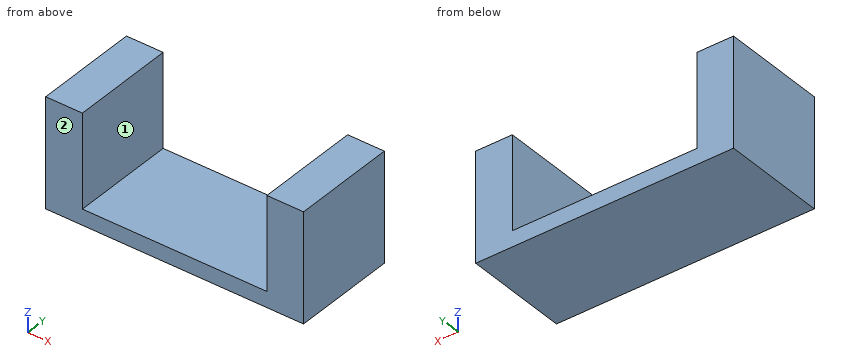
```python
from build123d import *

# Parameters (mm, degrees)
F0_W     = 54.864
F0_H     = 25.4
F1_DEPTH = 3.81
F2_W     = 5.08
F2_H     = 25.4
F3_DEPTH = 22.606
F5_W     = 25.4
F5_H     = 22.606
F5_H_2   = 3.81
F6_DEPTH = 3.81
F4_W     = 25.4
F4_H     = 3.81
F4_H_2   = 22.606
F7_DEPTH = 3.81


with BuildPart() as f1:
    # F0 (on Top) → F1 (new body)
    with BuildSketch(Plane.XY):
        Rectangle(F0_W, F0_H)
    extrude(amount=F1_DEPTH)

    # F2 (on face) → F3 (join)
    with BuildSketch(Plane.XY.offset(3.81)):
        with Locations((-24.892, 0)):
            Rectangle(F2_W, F2_H)
        with Locations((24.892, 0)):
            Rectangle(F2_W, F2_H)
    extrude(amount=F3_DEPTH)

    # F5 (on face) → F6 (join)
    with BuildSketch(Plane.YZ.offset(27.432)):
        with Locations((0, 11.303)):
            Rectangle(F5_W, F5_H)
        with Locations((0, 24.511)):
            Rectangle(F5_W, F5_H_2)
    extrude(amount=F6_DEPTH)

    # F4 (on face) → F7 (join)
    with BuildSketch(Plane(origin=(-27.432, 0, 0), x_dir=(0, -1, 0), z_dir=(-1, 0, 0))):
        with Locations((0, 24.511)):
            Rectangle(F4_W, F4_H)
        with Locations((0, 11.303)):
            Rectangle(F4_W, F4_H_2)
    extrude(amount=F7_DEPTH)


solid = f1.part
```
Check sheet for the modelled part. Datum: model origin and axes. Units: mm. Face numbers are marked on the shaded views. A direction names the side the tool comes from. Coordinates: 2 decimals unless noted, no trailing zeros. Loops run counter-clockwise (first coordinate to the right, second up) from the corner with the lowest first, then second, coordinate; pieces in that order, holes last. Notation, with made-up numbers: M -28.75,60.25 L -1.75,60.25 A31 ccw -1.75,88.25 Z; hole C 58,13 d8. An arc over 180 degrees is marked long. Answer as a JSON object with one key per item and string values.
1. Scan lines: L1, parallel to X at y = -5.75, z = 18; L2, parallel to Z at x = -16.5, y = 7. Record each from-to range of solid material in increasing order. Write a range as from..to.
Outcome:
{"L1": "-31.24..-22.35, 22.35..31.24", "L2": "0..3.81"}
2. Access from +Z, -Z, +X, -X, +Y, -Y to the whole of each face (thin tool, end or side, straight path). Record for the marked faces 1 and 2.
Outcome:
{"face 1": "+Z, +Y, -Y", "face 2": "+Z, -Z, +X, -X, -Y"}
3. Sectioned sample at A-A on z = 8. Record the cut outline in (x, y), and give its area (3 significant figures).
Outcome:
{"outline": "M -31.24,-12.7 L -22.35,-12.7 L -22.35,12.7 L -31.24,12.7 Z; M 22.35,-12.7 L 31.24,-12.7 L 31.24,12.7 L 22.35,12.7 Z", "area": "452 mm²"}
4. Depth check by flat-ended pin: P1, Ø12.5, axis at x = -3.5, y = -5, coming from the +Z side. Enter the tip coordinate at first touch or a pass-through.
Outcome:
{"P1": "z = 3.81"}
5. Sectioned sample at C-C on x = -14.5. Record the cut outline in (y, z), and give its area (3 significant figures).
Outcome:
{"outline": "M -12.7,0 L 12.7,0 L 12.7,3.81 L -12.7,3.81 Z", "area": "96.8 mm²"}
6. Sectioned sample at B-B on y = -1. Record the cut outline in (x, z), and give its area (3 significant figures).
Outcome:
{"outline": "M -31.24,0 L 31.24,0 L 31.24,26.42 L 22.35,26.42 L 22.35,3.81 L -22.35,3.81 L -22.35,26.42 L -31.24,26.42 Z", "area": "640 mm²"}
